Source: CAD feature listing. Evaluate the final solid. Frame: model axes, mm. Face numbers are marked on the shaded views. A direction names the side the tool comes from. Round coordinates to 2 decimals unless told otherwise and drop trailing zeros. Order: outer loops, then holes, each group sorted by start corner. A loop starts at its lowest first (then second) coordinate and runs counter-clockwise, first axis right, second up. Notation, with made-up numbers: (38.5, 25.25) - (80.5, 25.25) arc R17 ccw to (80.5, 34.25) - close; hole circle Ø5 at (22, 28). An arc over 180 degrees is marked (long way). Use one line per item in the form item = value. Start each with the question number.
Q1. Cut plane B-B, the plane y = -4. Return the cut outline in (x, z).
Q2. Pin query (flat end, axial travel): pin 1 Ø6 at (y, z) = (-9, 4.5) entering from -X; pin 2 Ø8 at (x, z) = (17.5, 19) entering from +Y; pin 3 Ø7.5 at (x, z) = (19, 3) entering from +Y; pin 4 Ø6 at (y, z) = (3, 23) entering from -X. Return the tip coordinate at first contact, or that it passes through.
Q3. Set-up query: the marked faces 1, 2 and 3. Return all of +Z, -Z, +X, -X, +Y, -Y with unobstructed straight access to the full face (end or side cutting, diameter ignored); none if empty.
Q4. Cut plane D-D, the plane y = -20.5. Return the cut outline in (x, z), and give its area (3 significant figures).
Q5. Cut plane A-A, the plane z = 0. Return the cut outline in (x, y), and give its area (3 significant figures).
Q6. Draft query along Y for the marked faces 4, 5 and 6. Return one class per face: released by +Y, released by -Y, zero draft, split by the parting line, or undercut.
Q7. Ray query, line 1 (Y direction, x = 13, z = 11); line 2 (X direction, y = 7.5, z = 13.5); line 3 (Z direction, x = 19.5, y = -20.5). Return the intervals inside material, ascending. Write a range as [from, to].
Q8. Cut plane C-C, the plane x = 20.25. Return the cut outline in (y, z), and give its area (3 significant figures).
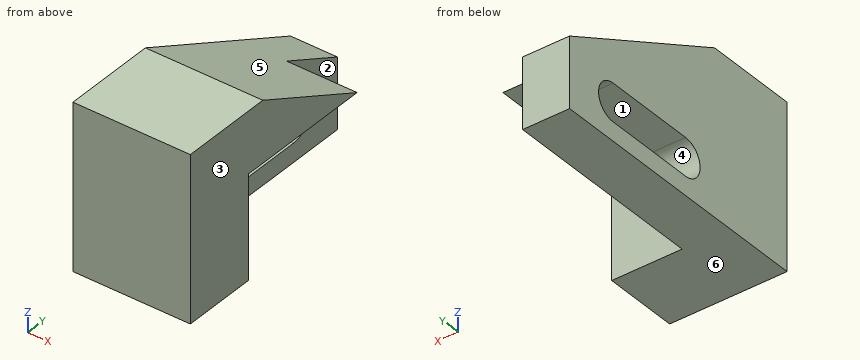
from build123d import *

# Parameters (mm, degrees)
BOSS_EXTRUDE1_DEPTH = 25
BOSS_EXTRUDE2_DEPTH = 25
CUT_EXTRUDE1_START  = 10
CUT_EXTRUDE1_DEPTH  = 15


with BuildPart() as part:
    # Sketch1 → Boss-Extrude1 (new body)
    with BuildSketch(Plane.YZ):
        Polygon((-38, 27), (-38, -8), (-22, -8), (-22, 14), (8, 14), (-18, 27), align=None)
    extrude(amount=BOSS_EXTRUDE1_DEPTH)

    # Sketch1<3> → Boss-Extrude2 (add)
    with BuildSketch(Plane.YZ):
        Polygon((-22, 14), (-22, -8), (22, -8), (22, 7), (8, 14), align=None)
        with BuildLine():
            ThreePointArc((-10, -4), (-14, 0), (-10, 4))
            Line((-10, 4), (10, 4))
            ThreePointArc((10, 4), (14, 0), (10, -4))
            Line((10, -4), (-10, -4))
        make_face(mode=Mode.SUBTRACT)
    extrude(amount=BOSS_EXTRUDE2_DEPTH)

    # Sketch1<4> → Cut-Extrude1 (cut)
    with BuildSketch(Plane.YZ.offset(CUT_EXTRUDE1_START)):
        Polygon((-22, 14), (-22, -8), (22, -8), (22, 7), (8, 14), align=None)
        with BuildLine():
            ThreePointArc((-10, -4), (-14, 0), (-10, 4))
            Line((-10, 4), (10, 4))
            ThreePointArc((10, 4), (14, 0), (10, -4))
            Line((10, -4), (-10, -4))
        make_face(mode=Mode.SUBTRACT)
    extrude(amount=CUT_EXTRUDE1_DEPTH, mode=Mode.SUBTRACT)


solid = part.part
Completed:
q1.outline = (0, -8) - (10, -8) - (10, -4) - (0, -4) - close; (0, 4) - (10, 4) - (10, 14) - (25, 14) - (25, 20) - (0, 20) - close
q2.pin_1 = 0
q2.pin_2 = 6
q2.pin_3 = -22
q2.pin_4 = through
q3.face_1 = +X, -X
q3.face_2 = -Z, +X, +Y
q3.face_3 = +Z, -Z, +X, +Y, -Y
q4.outline = (0, -8) - (10, -8) - (10, 14) - (25, 14) - (25, 27) - (0, 27) - close
q4.area = 545 mm2
q5.outline = (0, -38) - (25, -38) - (25, -22) - (10, -22) - (10, -14) - (0, -14) - close; (0, 14) - (10, 14) - (10, 22) - (0, 22) - close
q5.area = 560 mm2
q6.face_4 = undercut
q6.face_5 = released by +Y
q6.face_6 = zero draft
q7.line_1 = [-38, -22]
q7.line_2 = [0, 10]
q7.line_3 = [14, 27]
q8.outline = (-38, -8) - (-22, -8) - (-22, 14) - (8, 14) - (-18, 27) - (-38, 27) - close
q8.area = 781 mm2
